CAD build for the part. Positions are in the model's coordinates, mm. A direction names the side the tool comes from. Give positions to 0.01 mm unless a question says otherwise; leave off trailing zeros. Loops run counter-clockwise (first coordinate to the right, second up) from the corner with the lowest first, then second, coordinate; pieces in that order, holes last. Notation, with made-up numbers: (39, 82) - (81, 82) arc R18 ccw to (81, 103) - close; hole circle Ø4 at (-24, -18.5). An arc over 180 degrees is marked (long way). Return JSON: item names as keys, results as strings.
from build123d import *

# Parameters (mm, degrees)
F0_R     = 20
F1_DEPTH = 15
F2_R     = 18
F3_DEPTH = 13
F4_R     = 3.5
F4_R_2   = 1.5
F5_DEPTH = 16
F7_DEPTH = 2


with BuildPart() as f1:
    # F0 (on Top) → F1 (new body)
    with BuildSketch(Plane.XY):
        Circle(F0_R)
    extrude(amount=F1_DEPTH)

    # F2 (on face) → F3 (cut)
    with BuildSketch(Plane.XY.offset(15)):
        Circle(F2_R)
    extrude(amount=-F3_DEPTH, mode=Mode.SUBTRACT)

    # F4 (on face) → F5 (join)
    with BuildSketch(Plane.XY.offset(2)):
        Circle(F4_R)
        Circle(F4_R_2, mode=Mode.SUBTRACT)
    extrude(amount=F5_DEPTH)

    # F6 (on Top) → F7 (cut)
    with BuildSketch(Plane.XY):
        with BuildLine():
            Line((-13.61187, 5.615484), (-17.40644, 3.928479))
            ThreePointArc((-17.40644, 3.928479), (-17.844245, 0), (-17.40644, -3.928479))
            Line((-17.40644, -3.928479), (-13.61187, -5.615484))
            Line((-13.61187, -5.615484), (-3.885566, 0))
            Line((-3.885566, 0), (-13.61187, 5.615484))
        make_face()
        with BuildLine():
            Line((-11.669087, -8.980484), (-12.105382, -13.110179))
            ThreePointArc((-12.105382, -13.110179), (-8.922123, -15.45357), (-5.301057, -17.038658))
            Line((-5.301057, -17.038658), (-1.942783, -14.595968))
            Line((-1.942783, -14.595968), (-1.942783, -3.364999))
            Line((-1.942783, -3.364999), (-11.669087, -8.980484))
        make_face()
        with BuildLine():
            Line((1.942783, -14.595968), (5.301057, -17.038658))
            ThreePointArc((5.301057, -17.038658), (8.922123, -15.45357), (12.105382, -13.110179))
            Line((12.105382, -13.110179), (11.669087, -8.980484))
            Line((11.669087, -8.980484), (1.942783, -3.364999))
            Line((1.942783, -3.364999), (1.942783, -14.595968))
        make_face()
        with BuildLine():
            ThreePointArc((17.844245, 0), (17.734456, 1.976399), (17.40644, 3.928479))
            Line((17.40644, 3.928479), (13.61187, 5.615484))
            Line((13.61187, 5.615484), (3.885566, 0))
            Line((3.885566, 0), (13.61187, -5.615484))
            Line((13.61187, -5.615484), (17.40644, -3.928479))
            ThreePointArc((17.40644, -3.928479), (17.734456, -1.976399), (17.844245, 0))
        make_face()
        with BuildLine():
            ThreePointArc((12.105382, 13.110179), (8.922123, 15.45357), (5.301057, 17.038658))
            Line((5.301057, 17.038658), (1.942783, 14.595968))
            Line((1.942783, 14.595968), (1.942783, 3.364999))
            Line((1.942783, 3.364999), (11.669087, 8.980484))
            Line((11.669087, 8.980484), (12.105382, 13.110179))
        make_face()
        with BuildLine():
            Line((-11.669087, 8.980484), (-1.942783, 3.364999))
            Line((-1.942783, 3.364999), (-1.942783, 14.595968))
            Line((-1.942783, 14.595968), (-5.301057, 17.038658))
            ThreePointArc((-5.301057, 17.038658), (-8.922123, 15.45357), (-12.105382, 13.110179))
            Line((-12.105382, 13.110179), (-11.669087, 8.980484))
        make_face()
    extrude(amount=F7_DEPTH, mode=Mode.SUBTRACT)


solid = f1.part
1. Cut at A-A, the plane y = -7. Write the cut outline in (x, z) (3 decimals).
Values follow:
{"outline": "(-18.735, 0) - (-8.239, 0) - (-8.239, 2) - (-16.583, 2) - (-16.583, 15) - (-18.735, 15) - close; (-1.943, 0) - (1.943, 0) - (1.943, 2) - (-1.943, 2) - close; (8.239, 0) - (18.735, 0) - (18.735, 15) - (16.583, 15) - (16.583, 2) - (8.239, 2) - close"}
2. Pull direction X, two halves, no side cores. Call faces 1 (the face through (0, -2, 18)), 2 (the face through (8.874, -15.481, 0.986)): +X half, -X half, draft (parallel to the pull), parting line (faces both ways), or undercut.
Values follow:
{"face 1": "draft", "face 2": "undercut"}
3. Cut at D-D, the plane z = 1.5. Give the number of separate pieces and of enclosed holes in the cut face, plus the area to 3 significant figures.
Values follow:
{"separate pieces": "1", "enclosed holes": "6", "area": "698 mm²"}
4. Which spindle directions (+Z, -Z, +X, -X, +Y, -Y) get a long thin tool onto all of the face, cutting with end or side? Do faces 3 (the face through (-15, 5, 1)), 4 (the face through (3.233, -1.341, 9.888)). Say none if no direction does.
Values follow:
{"face 3": "+Z, -Z", "face 4": "+Z"}
5. Cut at C-C, the plane z = 14.5. Write the cut outline in (x, y).
Values follow:
{"outline": "circle Ø40 at (0, 0); circle Ø7 at (0, 0); hole circle Ø36 at (0, 0); hole circle Ø3 at (0, 0)"}
6. Drop flat-ended pins along their axis: P1, Ø1, axis at y = 11.5, z = 1, coming from the +X side; P2, Ø6, axis at x = 5, z = 5, coming from the -Y side; P3, Ø1, axis at x = 6, z = 4, coming from the +Y side. Give the stop position or say it passes through.
Values follow:
{"P1": "stops at x = 16.7", "P2": "stops at y = -19.9", "P3": "stops at y = 19.23"}
7. Cut at B-B, the plane x = 0. Write the cut outline in (y, z).
Values follow:
{"outline": "(-20, 0) - (20, 0) - (20, 15) - (18, 15) - (18, 2) - (3.5, 2) - (3.5, 18) - (1.5, 18) - (1.5, 2) - (-1.5, 2) - (-1.5, 18) - (-3.5, 18) - (-3.5, 2) - (-18, 2) - (-18, 15) - (-20, 15) - close"}
8. Drill centre lines: probe 1 along Y at (x, z) = (0, 6.75); probe 2 along Y at (x, z) = (-2.5, 6.5); probe 3 along X at (y, z) = (-8, 1). Where is each one in solid material? Low to high.
Values follow:
{"probe 1": "y = -20 to -18, -3.5 to -1.5, 1.5 to 3.5, 18 to 20", "probe 2": "y = -19.84 to -17.83, -2.45 to 2.45, 17.83 to 19.84", "probe 3": "x = -18.33 to -9.97, -1.94 to 1.94, 9.97 to 18.33"}
